```python
from build123d import *

# Parameters (mm, degrees)
SKETCH1_R           = 10
BOSS_EXTRUDE1_DEPTH = 15
SKETCH2_R           = 5
CUT_EXTRUDE1_DEPTH  = 5
BOSS_EXTRUDE2_DEPTH = 20
FILLET2_R           = 2


with BuildPart() as part:
    # Sketch1 → Boss-Extrude1 (new body)
    with BuildSketch(Plane(origin=(0, 0, 0), x_dir=(1, 0, 0), z_dir=(0, 1, 0))):
        with Locations(Location((-10.491071429, 0.647321429, 0), (0, 0, 270))):
            Circle(SKETCH1_R)
    extrude(amount=BOSS_EXTRUDE1_DEPTH)

    # Sketch2 → Cut-Extrude1 (cut)
    with BuildSketch(Plane(origin=(0, 15, 0), x_dir=(1, 0, 0), z_dir=(0, 1, 0))):
        with Locations(Location((-10.491071429, 0.647321429, 0), (0, 0, 270))):
            Circle(SKETCH2_R)
    extrude(amount=-CUT_EXTRUDE1_DEPTH, mode=Mode.SUBTRACT)

    # Sketch3 → Boss-Extrude2 (add)
    with BuildSketch(Plane(origin=(0, 0, 0), x_dir=(-1, 0, 0), z_dir=(0, -1, 0))):
        Polygon((8.015436801, 2.132099703), (7.96739841, -0.754251912), (10.443033038, -2.239030187), (12.966706056, -0.837456846), (13.014744447, 2.04889477), (10.539109819, 3.533673044), align=None)
    extrude(amount=BOSS_EXTRUDE2_DEPTH)

    # Fillet2
    fillet2_edges = [part.edges().sort_by_distance(p)[0] for p in [
        (-9.27727331, 0, -2.832886373),
        (-7.991417606, 0, -0.688923895),
        (-9.205215724, 0, 1.496641049),
        (-11.704869547, 0, 1.538243516),
        (-12.990725252, 0, -0.605718962),
        (-11.776927133, 0, -2.791283907),
    ]]
    fillet(fillet2_edges, radius=FILLET2_R)


solid = part.part
```
The model under review builds one solid part; all positions refer to its coordinate system, in mm. A direction names the side the tool comes from. Give positions to 0.01 mm unless a question says otherwise; leave off trailing zeros. Write each loop counter-clockwise with the first axis right and the second up, starting at its lowest first coordinate (ties: lowest second). Pieces come first, ordered by that corner, then holes.
(1) For P1, Ø1, axis at x = -11, z = -5.5, coming from the -Y side; P2, Ø4, axis at y = -6, z = 0, coming from the -X side; P3, Ø2, axis at x = -13.5, z = -3, coming from the +Y side, all flat-tipped, find the tip position at first contact; note any pin that passes through.
(2) Consider section D-D, the plane z = -8. Give the boundary of the cut face in (x, y).
(3) The part is to be moulded in two halves that separate along Z. For faces 6 (the cylindrical face through (-10.271, 12.535, -5.642)), 7 (the cylindrical face through (-8.823, -0.349, -3.577)), 8 (the flat face through (-10, -20, -1)), say which applies: released by +Z, released by -Z, zero draft, split by the parting line, or undercut.
(4) To check wall thickness, follow L1, parallel to Y at x = -13.5, z = -7.25; L2, parallel to X at y = -16.5, z = 0.25; L3, parallel to Y at x = -9.5, z = -2.25. State the ranges of each line that lie inside material, in increasing order.
(5) Consider section C-C, the plane x = -2. Give the boundary of the cut face in (y, z), and give its area (3 significant figures).
(6) Consider section B-B, the plane y = 11.5. Give the boundary of the cut face in (x, z).
(7) Tool access review of faces 1 (the flat face through (-11.794, -10.874, -2.781)), 2 (the flat face through (-9.29, -10.87, -2.84)), 3 (the flat face through (-9.188, -10.874, 1.486)), 4 (the flat face through (-13, 0, 4)), 5 (the flat face through (-10, 10, -1)): name each direction out of +Z, -Z, +X, -X, +Y, -Y from which nothing blocks a thin tool from reaching the whole face with its end or side.
(8) Consider section A-A, the plane y = -7.5. Give the boundary of the cut face in (x, z).
Returned:
1. P1: stops at y = -0.08
1. P2: stops at x = -13.01
1. P3: stops at y = 10
2. outline: (-17.27, 0) - (-3.71, 0) - (-3.71, 15) - (-17.27, 15) - close
3. face 6: undercut
3. face 7: released by -Z
3. face 8: zero draft
4. L1: y = 0 to 15
4. L2: x = -12.98 to -7.98
4. L3: y = -20 to 10
5. outline: (0, -5.93) - (15, -5.93) - (15, 4.63) - (0, 4.63) - close
5. area: 158 mm2
6. outline: circle Ø20 at (-10.49, -0.65); hole circle Ø10 at (-10.49, -0.65)
7. face 1: -Z, -X, -Y
7. face 2: -Z, +X, -Y
7. face 3: +Z, +X, -Y
7. face 4: -Y
7. face 5: +Y
8. outline: (-13.01, -2.05) - (-10.54, -3.53) - (-8.02, -2.13) - (-7.97, 0.75) - (-10.44, 2.24) - (-12.97, 0.84) - close
